Build history of the part. All positions in model axes, mm. A direction names the side the tool comes from. Coordinates: 2 decimals unless noted, no trailing zeros. Order: outer loops, then holes, each group sorted by start corner. A loop starts at its lowest first (then second) coordinate and runs counter-clockwise, first axis right, second up. Notation, with made-up numbers: M 43.5,69 L 48.5,69 A16 cw 48.5,85 Z; hole C -33,8 d10. An arc over 180 degrees is marked long. Use a Markdown table: item, result. Add a question column.
from build123d import *

# Parameters (mm, degrees)
SKETCH3_W           = 100
SKETCH3_H           = 50
SKETCH3_W_2         = 40
SKETCH3_H_2         = 3
SKETCH3_W_3         = 3
SKETCH3_H_3         = 10
SKETCH3_W_4         = 60
SKETCH3_H_4         = 20
BOSS_EXTRUDE2_DEPTH = 3


with BuildPart() as part:
    # Sketch3 → Boss-Extrude2 (new body)
    with BuildSketch(Plane.XY):
        Rectangle(SKETCH3_W, SKETCH3_H)
        with Locations((0, -21.5)):
            Rectangle(SKETCH3_W_2, SKETCH3_H_2, mode=Mode.SUBTRACT)
        with Locations((-46.5, 15)):
            Rectangle(SKETCH3_W_3, SKETCH3_H_3, mode=Mode.SUBTRACT)
        Rectangle(SKETCH3_W_4, SKETCH3_H_4, mode=Mode.SUBTRACT)
        with Locations((46.5, 15)):
            Rectangle(SKETCH3_W_3, SKETCH3_H_3, mode=Mode.SUBTRACT)
        with Locations((46.5, -15)):
            Rectangle(SKETCH3_W_3, SKETCH3_H_3, mode=Mode.SUBTRACT)
        with Locations((-46.5, -15)):
            Rectangle(SKETCH3_W_3, SKETCH3_H_3, mode=Mode.SUBTRACT)
    extrude(amount=BOSS_EXTRUDE2_DEPTH)


solid = part.part
(1) Which spindle directions (+Z, -Z, +X, -X, +Y, -Y) get a long thin tool onto all of the face, cutting with end or side? Do faces 4 (the flat face through (50, 0, 1)), 5 (the flat face through (48, -15, 1)). Say none if no direction does.
(2) Slice it at C-C on x = -25. Give the cut face in (y, z), and give its area (3 significant figures).
(3) Mould opens along Y. For faces 1 (the flat face through (-1, -25, 1)), 2 (the flat face through (-47, 20, 1)), 3 (the flat face through (-1, 25, 1)) say: released by +Y, released by -Y, zero draft, split by the parting line, or undercut.
(4) Slice it at D-D on z = 1. Give the cut face in (x, y).
(5) Slice it at B-B on y = -3. Give the cut face in (x, z), and give its area (3 significant figures).
(6) Drill centre lines: line 1 along X through (y, z) = (15.5, 1); line 2 along Y through (x, z) = (-15, 0.9); line 3 along X through (y, z) = (-7.5, 1.45). Where is each one in solid material? Low to high. Write a range as from..to.
(7) Slice it at A-A on x = -14. Give the cut face in (y, z), and give its area (3 significant figures).
Solutions:
| question | item | result |
|---|---|---|
| 1 | face 4 | +Z, -Z, +X, +Y, -Y |
| 1 | face 5 | +Z, -Z |
| 2 | outline | M -25,0 L -10,0 L -10,3 L -25,3 Z; M 10,0 L 25,0 L 25,3 L 10,3 Z |
| 2 | area | 90.0 mm² |
| 3 | face 1 | released by -Y |
| 3 | face 2 | undercut |
| 3 | face 3 | released by +Y |
| 4 | outline | M -50,-25 L 50,-25 L 50,25 L -50,25 Z; hole M -48,-20 L -45,-20 L -45,-10 L -48,-10 Z; hole M -48,10 L -45,10 L -45,20 L -48,20 Z; hole M -30,-10 L 30,-10 L 30,10 L -30,10 Z; hole M -20,-23 L 20,-23 L 20,-20 L -20,-20 Z; hole M 45,-20 L 48,-20 L 48,-10 L 45,-10 Z; hole M 45,10 L 48,10 L 48,20 L 45,20 Z |
| 5 | outline | M -50,0 L -30,0 L -30,3 L -50,3 Z; M 30,0 L 50,0 L 50,3 L 30,3 Z |
| 5 | area | 120 mm² |
| 6 | line 1 | -50..-48, -45..45, 48..50 |
| 6 | line 2 | -25..-23, -20..-10, 10..25 |
| 6 | line 3 | -50..-30, 30..50 |
| 7 | outline | M -25,0 L -23,0 L -23,3 L -25,3 Z; M -20,0 L -10,0 L -10,3 L -20,3 Z; M 10,0 L 25,0 L 25,3 L 10,3 Z |
| 7 | area | 81.0 mm² |
